Can you work these out from the model? Positions are in its coordinate system, mm. A direction names the side the tool comes from. Give positions to 0.01 mm unless a question says otherwise; leave off trailing zeros. Write each loop counter-clockwise with the first axis right and the second up, starting at its lowest first coordinate (ties: lowest second). Pieces come first, ordered by that corner, then holes. Notation, with made-up numbers: (8, 80) -> (29, 80) arc R18 cw to (29, 98) -> close; hole circle Ø2 at (-27, -18). An arc over 180 degrees is marked (long way). Answer as CSV lines item,"result". Start each with the question number.
1. I'm going to push flat-ended pins straight in: P1, Ø1, axis at y = 1.5, z = 1, coming from the -X side; P2, Ø1.5, axis at y = 1, z = -1, coming from the +X side; P3, Ø1, axis at x = -0.5, y = 1.5, coming from the -Z side (3 decimals). Where does each tip first touch, or does it pass through?
2. If we section it at A-A on y = 0.6: Write out the boundary of the cut face in (x, z).
3. If we mould it in two halves opening along Z, with no side actions, what happens to faces 3 (the face through (0.082, 1.366, -1.873)), 4 (the face through (0.45, 0.61, 1.43)), 5 (the face through (-1.3, -0.75, 1.3))? For each: pulls with the +Z half, pulls with the -Z half, needs draft (parallel to the pull), parting line crosses it, or undercut.
4. On a 3-axis mill with a long thin cutter (end or side, diameter ignored), from which of +Z, -Z, +X, -X, +Y, -Y can I reach the whole of each face in a straight line? I mean faces 1 (the face through (-2, 0.75, 1)), 2 (the face through (-1.15, 0.04, 2.77)). Say none if no direction works.
5. If we section it at B-B on y = 0.95: Write out the boundary of the cut face in (x, z) (3 decimals).
6. I need wall thicknesses on line 1 (Z direction, x = 0, y = 0.7); line 2 (X direction, y = 1.45, z = 0) (3 decimals). Which ranges of each line are inside material? Lowest first, please. Write a range as [from, to].
```python
from build123d import *

# Parameters (mm, degrees)
SKETCH1_R               = 3
BOSS_EXTRUDE1_DEPTH     = 0.75
BOSS_EXTRUDE2_START     = 0.75
SKETCH1_3_R             = 1.875
BOSS_EXTRUDE2_DEPTH     = 1.25
CUT_EXTRUDE1_DEPTH      = 5.69041576
CUT_EXTRUDE1_DEPTH_BACK = 5.69041576
SKETCH1_4_R             = 1.5
CIRPATTERN1_COUNT       = 4
CHAMFER1_SIZE           = 0.062


with BuildPart() as part:
    # Sketch1 → Boss-Extrude1 (new, symmetric)
    with BuildSketch(Plane(origin=(0, 0, 0), x_dir=(1, 0, 0), z_dir=(0, 1, 0))):
        with Locations(Location((0, 0, 0), (0, 0, 270))):
            Circle(SKETCH1_R)
    extrude(amount=BOSS_EXTRUDE1_DEPTH, both=True)

    # Sketch1_3 → Boss-Extrude2 (add)
    with BuildSketch(Plane(origin=(0, 0, 0), x_dir=(1, 0, 0), z_dir=(0, 1, 0)).offset(BOSS_EXTRUDE2_START)):
        with Locations(Location((0, 0, 0), (0, 0, 270))):
            Circle(SKETCH1_3_R)
    extrude(amount=BOSS_EXTRUDE2_DEPTH)

    # Sketch1_4 → Cut-Extrude1 (cut, two sides: drawn at the far end of the back side and taken through both)
    with BuildSketch(Plane(origin=(0, 0, 0), x_dir=(1, 0, 0), z_dir=(0, 1, 0)).offset(-CUT_EXTRUDE1_DEPTH_BACK)):
        with Locations(Location((0, 0, 0), (0, 0, 270))):
            Circle(SKETCH1_4_R)
    extrude(amount=CUT_EXTRUDE1_DEPTH + CUT_EXTRUDE1_DEPTH_BACK, mode=Mode.SUBTRACT)

    # Sketch4 → 1.0mm Dowel Hole1 (revolve, cut)
    with BuildSketch(Plane(origin=(0.046321233, 0, 2.999642369), x_dir=(0.999880789746526, 0, -0.015440411129998149), z_dir=(0, 1, 0))):
        Polygon((0, 0), (0, 1.525022302), (0.3745, 1.3), (0.3745, 0), align=None)
    f_1_0mm_dowel_hole1 = revolve(axis=Axis((0.144367844, 0, 9.348885384), (-0.015440411129998149, 0, -0.999880789746526)), mode=Mode.SUBTRACT)

    # CirPattern1: 1.0mm Dowel Hole1 ×4 about axis
    cirpattern1_axis = Axis((0, 0.75, 0), (0, 1, 0))
    for i in range(1, CIRPATTERN1_COUNT):
        add(f_1_0mm_dowel_hole1.rotate(cirpattern1_axis, i * 360 / CIRPATTERN1_COUNT), mode=Mode.SUBTRACT)

    # Chamfer1
    chamfer1_edges = [part.edges().sort_by_distance(p)[0] for p in [
        (0, -0.75, -3),
    ]]
    chamfer(chamfer1_edges, length=CHAMFER1_SIZE)


solid = part.part
```
Computed values:
1,P1,"stops at x = -1.81"
1,P2,"stops at x = 2.99"
1,P3,"stops at z = -1.875"
2,outline,"circle Ø6 at (0, 0); hole circle Ø3 at (0, 0)"
3,face 3,"parting line crosses it"
3,face 4,"undercut"
3,face 5,"needs draft"
4,face 1,"+Y"
4,face 2,"+Y, -Y"
5,outline,"circle Ø3.75 at (0, 0); hole circle Ø3 at (0, 0)"
6,line 1,"z = [-3, -1.5], [1.5, 3]"
6,line 2,"x = [-1.875, -1.5], [1.5, 1.875]"
